For this review, take the finished solid that the model builds, in its own axes (mm). Coordinates: 2 decimals unless noted, no trailing zeros. Write each loop counter-clockwise with the first axis right and the second up, starting at its lowest first coordinate (ties: lowest second). Pieces come first, ordered by that corner, then holes. Notation, with made-up numbers: (84.5, 63.5) -> (92.5, 63.5) arc R16 cw to (92.5, 75.5) -> close; hole circle Ø11 at (-37, -25.5). An arc over 180 degrees is marked (long way). Put each result on its own line as item: value. Start each with the question number.
Item 1: Insertion check: P1, Ø2, axis at y = 24.5, z = 2.5, coming from the -X side; P2, Ø2, axis at y = 37, z = 3.5, coming from the +X side; P3, Ø2, axis at x = -0.5, z = 4, coming from the +Y side. Each pin has a flat end and moves straight along its axis. Give the tip position at first contact, or say it passes through.
Item 2: Consider section C-C on x = 39.5. Give the boundary of the cut face in (y, z).
Item 3: To check wall thickness, follow L1, parallel to X at y = 54.5, z = 0.5; L2, parallel to X at y = 68, z = 4.75; L3, parallel to X at y = 18.5, z = 0.75. State the ranges of each line that lie inside material, in increasing order.
Item 4: Consider section D-D on z = 3.25. Give the number of separate pieces and of enclosed holes in the cut face, and give its area (3 significant figures).
Item 5: Consider section B-B on x = 20. Give the boundary of the cut face in (y, z), and give its area (3 significant figures).
Item 6: Consider section A-A on y = 17.5. Give the boundary of the cut face in (x, z).
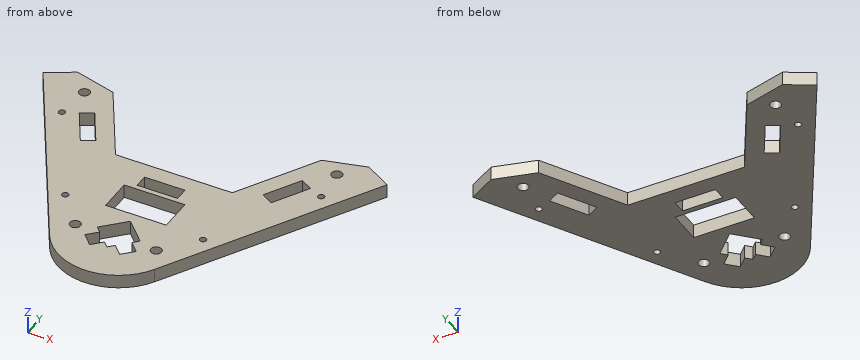
Autodesk Inventor part; units mm, degrees
ref_plane "YZ Plane" through (0, 0, 0) normal (1, 0, 0) x (0, 1, 0)
ref_plane "XZ Plane" through (0, 0, 0) normal (0, 1, 0) x (-1, 0, 0)
ref_plane "XY Plane" through (0, 0, 0) normal (0, 0, 1) x (1, 0, 0)
sketch "Sketch1" plane through (0, 0, 0) normal (0, 0, 1) x (1, 0, 0)
  line L0 (-10.6066, 0) -> (0, 10.6066)
  line L1 (0, 10.6066) -> (10.6066, 0)
  line L2 (10.6066, 0) -> (0, -10.6066)
  line L3 (0, -10.6066) -> (-10.6066, 0)
  arc A0 (-25.9808, -15) -> (25.9808, -15) centre (0, 0) ccw
  line L4 (25.9808, -15) -> (85, 87.2243)
  line L5 (10, 41.731) -> (10, 35)
  line L6 (10, 35) -> (-10, 35)
  line L7 (-10, 35) -> (-10, 41.731)
  line L8 (-10, 41.731) -> (10, 41.731)
  line L9 (-85, 87.2243) -> (-25.9808, -15)
  circle A1 centre (-49.0748, 40) radius 1.6
  circle A2 centre (-64.0748, 65.9808) radius 1.6
  circle A3 centre (49.0748, 40) radius 1.6
  circle A4 centre (64.0748, 65.9808) radius 1.6
  line L10 (-85, 87.2243) -> (-72.0096, 94.7243)
  line L11 (-51.5192, 89.2339) -> (-28.8675, 50)
  line L12 (-28.8675, 50) -> (28.8675, 50)
  line L13 (28.8675, 50) -> (51.5192, 89.2339)
  line L14 (2.6517, -7.955) -> (7.955, -2.6517)
  line L15 (7.955, -2.6517) -> (12.7145, -7.4112)
  line L16 (12.7145, -7.4112) -> (7.4112, -12.7145)
  line L17 (7.4112, -12.7145) -> (2.6517, -7.955)
  line L18 (-2.6517, -7.955) -> (-7.4112, -12.7145)
  line L19 (-7.4112, -12.7145) -> (-12.7145, -7.4112)
  line L20 (-12.7145, -7.4112) -> (-7.955, -2.6517)
  line L21 (-7.955, -2.6517) -> (-2.6517, -7.955)
  circle A5 centre (-37.3546, 40) radius 2.65
  circle A6 centre (37.3546, 40) radius 2.65
  circle A7 centre (-62.3546, 83.3013) radius 2.65
  circle A8 centre (62.3546, 83.3013) radius 2.65
  circle A9 centre (-20, -2.65) radius 2.65
  circle A10 centre (20, -2.65) radius 2.65
  line L22 (-57.1495, 68.9859) -> (-47.1495, 51.6654)
  line L23 (-47.1495, 51.6654) -> (-41.3203, 55.0309)
  line L24 (-41.3203, 55.0309) -> (-51.3203, 72.3514)
  line L25 (-51.3203, 72.3514) -> (-57.1495, 68.9859)
  line L26 (47.1495, 51.6654) -> (57.1495, 68.9859)
  line L27 (57.1495, 68.9859) -> (51.3203, 72.3514)
  line L28 (51.3203, 72.3514) -> (41.3203, 55.0309)
  line L29 (41.3203, 55.0309) -> (47.1495, 51.6654)
  line L30 (-15, 32.5) -> (15, 32.5)
  line L31 (15, 32.5) -> (15, 15.6066)
  line L32 (15, 15.6066) -> (-15, 15.6066)
  line L33 (-15, 15.6066) -> (-15, 32.5)
  line L34 (-10.6066, 0) -> (10.6066, 0)
  line L35 (25.9808, -15) -> (0, -60)
  line L36 (0, -60) -> (-25.9808, -15)
  line L37 (85, 87.2243) -> (72.0096, 94.7243)
  circle A11 centre (-34.0748, 14.0192) radius 1.6
  circle A12 centre (34.0748, 14.0192) radius 1.6
  line L38 (72.0096, 94.7243) -> (51.5192, 89.2339)
  line L39 (-51.5192, 89.2339) -> (-72.0096, 94.7243)
  point P0 (0, 0)
  point P1 (0, 35)
  point P2 (0, 32.5)
  dimension "d0" = 15
  dimension "d9" = 30
  dimension "d11" = 6.731
  dimension "d12" = 20
  dimension "d25" = 60
  dimension "d34" = 3.2
  dimension "d36" = 30
  dimension "d38" = 30
  dimension "d40" = 7.5
  dimension "d41" = 7.5
  dimension "d42" = 7.5
  dimension "d43" = 7.5
  dimension "d45" = 40
  dimension "d54" = 50
  dimension "d55" = 0
  dimension "d56" = 0
  dimension "d57" = 7.5
  dimension "d58" = 3.75
  dimension "d63" = 15
  dimension "d64" = 5.3
  dimension "d66" = 50
  dimension "d67" = 15
  dimension "d68" = 15
  dimension "d73" = 20
  dimension "d74" = 15
  dimension "d75" = 15
  dimension "d76" = 15
  dimension "d77" = 15
  dimension "d79" = 35
  dimension "d80" = 2.5
  dimension "d81" = 5
  dimension "d82" = 30
  dimension "d83" = 20
  dimension "d84" = 20
  dimension "d85" = 40
  dimension "d86" = 170
  dimension "d88" = 30
  dimension "d89" = 30
  dimension "d90" = 7.5
  dimension "d91" = 7.5
  dimension "d92" = 135
  dimension "d93" = 30
  dimension "d94" = 45
  dimension "d95" = 15
extrude "Extrusion2" add sketch "Sketch1" along normal blind 6.731 contours L9 L10 L39 L11 L12 L13 L38 L37 L4 A0 | A5 | A6
sketch "Sketch2" plane through (0, 0, 6.731) normal (0, 0, 1) x (1, 0, 0)
  circle A0 centre (49.0748, 40) radius 1.6
  circle A1 centre (-49.0748, 40) radius 1.6
extrude "Extrusion3" add sketch "Sketch2" against normal up to surface (6.731 mm away)
equation "\"d38\" = d36"
equation "\"d41\" = d40"
equation "\"d58\" = 0.5 * d57"
equation "\"THICKA\" = 3.175"
equation "\"THICKB\" = 6.731"
equation "\"THICKC\" = 12.7"
equation "\"BALLDIA\" = 12"
equation "\"MAGDIA\" = 9.5"
equation "\"THICKPLY\" = 5"
properties part number "Frame_Lower_Plate_Bottom"
Return value:
1. P1: x = -49.36
1. P2: x = 56.58
1. P3: y = 50
2. outline: (8.42, 0) -> (68.42, 0) -> (68.42, 6.73) -> (8.42, 6.73) -> close
3. L1: -66.11 to -48.79, -42.24 to -31.47, 31.47 to 42.24, 48.79 to 66.11
3. L2: -73.9 to -56.58, -48.81 to -39.26, 39.26 to 48.81, 56.58 to 73.9
3. L3: -45.32 to -15, 15 to 45.32
4. separate pieces: 1
4. enclosed holes: 13
4. area: 7,890 mm^2
5. outline: (-22.36, 0) -> (-5.3, 0) -> (-5.3, 6.73) -> (-22.36, 6.73) -> close; (0, 0) -> (50, 0) -> (50, 6.73) -> (0, 6.73) -> close
5. area: 451 mm^2
6. outline: (-44.74, 0) -> (-15, 0) -> (-15, 6.73) -> (-44.74, 6.73) -> close; (15, 0) -> (44.74, 0) -> (44.74, 6.73) -> (15, 6.73) -> close
